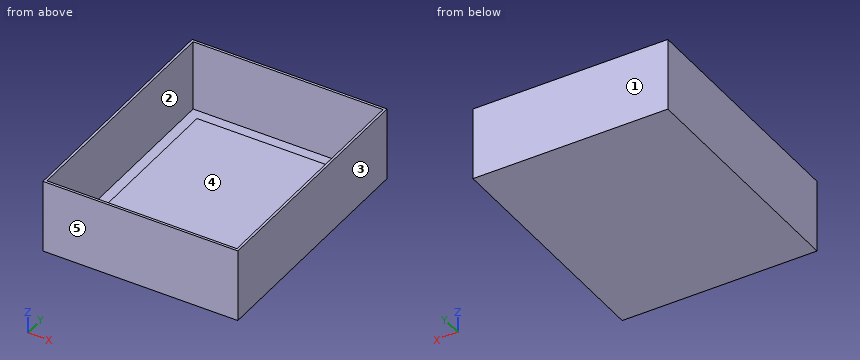
```python
from build123d import *

# Parameters (mm, degrees)
SKETCH1_W           = 406.4
SKETCH1_H           = 508
BOSS_EXTRUDE1_DEPTH = 152.4
SHELL1_T            = -5.08
SKETCH2_W           = 350.52
SKETCH2_H           = 449.58
BOSS_EXTRUDE2_DEPTH = 2.54


with BuildPart() as part:
    # Sketch1 → Boss-Extrude1 (new body)
    with BuildSketch(Plane.XY):
        Rectangle(SKETCH1_W, SKETCH1_H)
    extrude(amount=BOSS_EXTRUDE1_DEPTH)

    # Shell1
    shell1_openings = [part.faces().sort_by_distance(p)[0] for p in [
        (0, 0, 152.4),
    ]]
    offset(amount=SHELL1_T, openings=shell1_openings, kind=Kind.INTERSECTION)

    # Sketch2 → Boss-Extrude2 (add)
    with BuildSketch(Plane.XY.offset(5.08)):
        Rectangle(SKETCH2_W, SKETCH2_H)
    extrude(amount=BOSS_EXTRUDE2_DEPTH)


solid = part.part
```
Part model, mm, in its own coordinate system. Face numbers are marked on the shaded views. A direction names the side the tool comes from. Give positions to 0.01 mm unless a question says otherwise; leave off trailing zeros. Order: outer loops, then holes, each group sorted by start corner. A loop starts at its lowest first (then second) coordinate and runs counter-clockwise, first axis right, second up. Notation, with made-up numbers: M -16.75,13 L -1.75,13 A25 ccw -1.75,30 Z; hole C 8.25,-24 d9. An arc over 180 degrees is marked long. Use a Markdown table: item, result. Add a question column.
(1) Mould opens along X. For the marked faces 3, 4 and 5 say: +X half, -X half, draft (parallel to the pull), parting line (faces both ways), or undercut.
(2) Probe line 1 along X through (y, z) = (202, 41.5); line 2 along Y through (x, z) = (51, 16); line 3 along Z through (x, y) = (-98, 76). List the from-to ranges inside material, lowest first. Write a range as [from, to].
(3) 3-axis set-ups, long thin cutter, end or side, ignore diameter. For the marked faces 1 and 2: which of +Z, -Z, +X, -X, +Y, -Y reach the whole face in a straight line?
(4) Saw through at B-B, the plane y = -143.5. Give the cut face in (x, z), and give its area (3 significant figures).
(5) Saw through at C-C, the plane x = 130.5. Give the cut face in (y, z), and give its area (3 significant figures).
(6) Saw through at A-A, the plane z = 93. Give the cut face in (x, y).
(7) Drop a flat-ended pin along its axis: P1, Ø5, axis at x = 135.5, y = 127, coming from the +Z side. Give the stop position or say it passes through.
Answer key:
| question | item | result |
|---|---|---|
| 1 | face 3 | +X half |
| 1 | face 4 | undercut |
| 1 | face 5 | draft |
| 2 | line 1 | [-203.2, -198.12], [198.12, 203.2] |
| 2 | line 2 | [-254, -248.92], [248.92, 254] |
| 2 | line 3 | [0, 7.62] |
| 3 | face 1 | +Z, -Z, +X, -X, +Y |
| 3 | face 2 | +Z |
| 4 | outline | M -203.2,0 L 203.2,0 L 203.2,152.4 L 198.12,152.4 L 198.12,5.08 L 175.26,5.08 L 175.26,7.62 L -175.26,7.62 L -175.26,5.08 L -198.12,5.08 L -198.12,152.4 L -203.2,152.4 Z |
| 4 | area | 4,450 mm^2 |
| 5 | outline | M -254,0 L 254,0 L 254,152.4 L 248.92,152.4 L 248.92,5.08 L 224.79,5.08 L 224.79,7.62 L -224.79,7.62 L -224.79,5.08 L -248.92,5.08 L -248.92,152.4 L -254,152.4 Z |
| 5 | area | 5,220 mm^2 |
| 6 | outline | M -203.2,-254 L 203.2,-254 L 203.2,254 L -203.2,254 Z; hole M -198.12,-248.92 L 198.12,-248.92 L 198.12,248.92 L -198.12,248.92 Z |
| 7 | P1 | z = 7.62 |
